Check sheet for the drawn part. Datum: minimum x, y, z corner. Units: mm. A direction names the side the tool comes from. Give positions to 0.01 mm unless a question says otherwise; leave off trailing zeros. Write each loop counter-clockwise with the first axis right and the second up, starting at its lowest first coordinate (ties: lowest second). Pieces come first, ordered by that corner, then holes. Notation, with made-up numbers: (3.5, 81.5) - (33.5, 81.5) arc R23 cw to (33.5, 105.5) - close; hole circle Ø6 at (78, 34). An arc over 180 degrees is marked (long way). One line per question, with ' | ' between items. Start each with the question number.
Q1. Gauge pin test, flat ends, axial feed: P1, Ø7.5, axis at x = 25, z = 7, coming from the +Y side; P2, Ø2, axis at x = 16.5, y = 5.5, coming from the -Z side; P3, Ø6, axis at x = 11, z = 6.5, coming from the -Y side; P4, Ø1.9, axis at x = 57, y = 3.16, coming from the -Z side. Record the tip position at first contact, or that the pin passes through.
Q2. Section check B-B on z = 11. Record the boundary of the cut face in (x, y), and give its area (3 significant figures).
Q3. Thickness scan on L1, parallel to X at y = 3.25, z = 10; L2, parallel to Y at x = 57, z = 8.25; L3, parallel to Y at x = 6, z = 7.7. Record the ranges inside material, lowest first. Write a range as [from, to].
Q4. Section check D-D on x = 18. Record the boundary of the cut face in (y, z).
Q5. Release check for a two-part mould opening along X. For the marked faces 1, 2 and 3 record: +X half, -X half, draft (parallel to the pull), parting line (faces both ways), or undercut.
Q6. Set-up check for the marked faces 4, 5 and 6: record each of +Z, -Z, +X, -X, +Y, -Y from which the full face is reachable in a straight line by a thin tool's end or side.
Q7. Section check C-C on z = 2. Record the boundary of the cut face in (x, y), and give its area (3 significant figures).
Q8. Section check A-A on x = 56. Record the boundary of the cut face in (y, z).
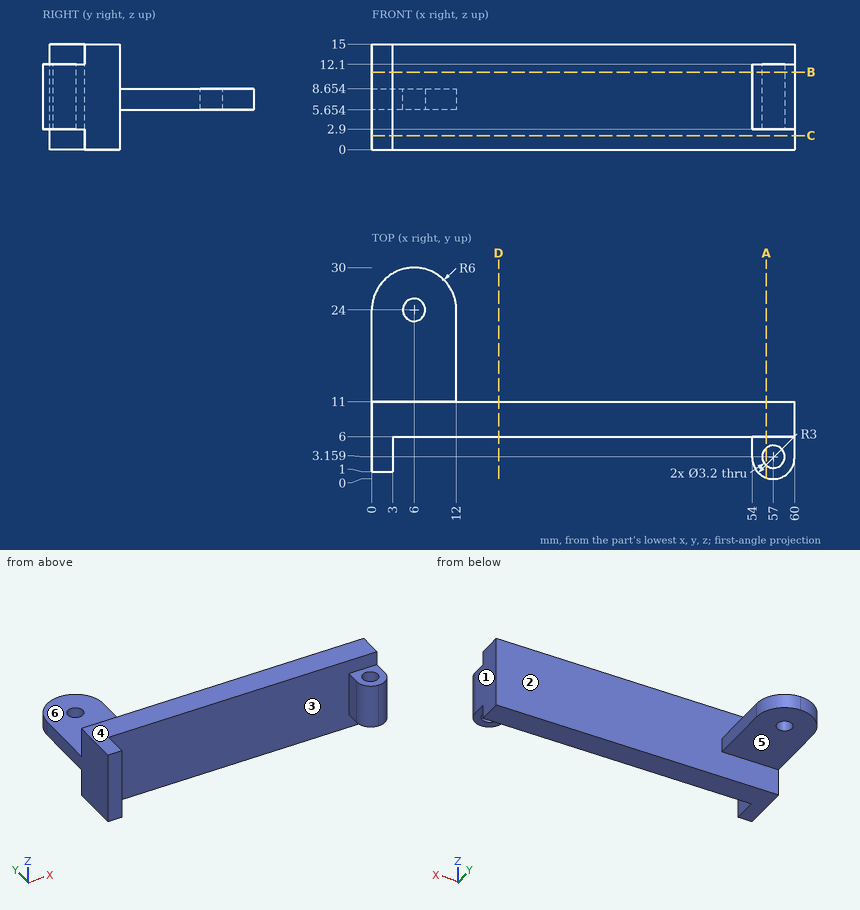
Working result:
1) P1: stops at y = 11 | P2: stops at z = 0 | P3: stops at y = 6 | P4: passes through
2) outline: (0, 1) - (3, 1) - (3, 6) - (54, 6) - (54, 3) arc R3 ccw to (60, 3) - (60, 11) - (0, 11) - close; hole circle Ø3.2 at (57, 3.16) | area: 339 mm2
3) L1: x = [0, 3], [54, 55.4], [58.6, 60] | L2: y = [0, 1.56], [4.76, 11] | L3: y = [6, 22.4], [25.6, 30]
4) outline: (6, 0) - (11, 0) - (11, 15) - (6, 15) - close
5) face 1: +X half | face 2: draft | face 3: undercut
6) face 4: +Z, +X, -X, +Y, -Y | face 5: -Z, +X, -X, +Y | face 6: +Z, +X, -X, +Y
7) outline: (0, 1) - (3, 1) - (3, 6) - (60, 6) - (60, 11) - (0, 11) - close | area: 315 mm2
8) outline: (0.17, 2.9) - (1.91, 2.9) - (1.91, 12.1) - (0.17, 12.1) - close; (4.41, 2.9) - (6, 2.9) - (6, 0) - (11, 0) - (11, 15) - (6, 15) - (6, 12.1) - (4.41, 12.1) - close
